Read the model definition and answer for the solid it produces. Units are mm, in the model's axes. Give positions to 0.01 mm unless a question says otherwise; leave off trailing zeros. Loops run counter-clockwise (first coordinate to the right, second up) from the corner with the lowest first, then second, coordinate; pieces in that order, holes last. Notation, with made-up numbers: (69.25, 17) - (108.25, 17) arc R20 cw to (108.25, 27) - close; hole circle Ø10 at (79, 67.25). An arc over 180 degrees is marked (long way). Write item = value, one per line.
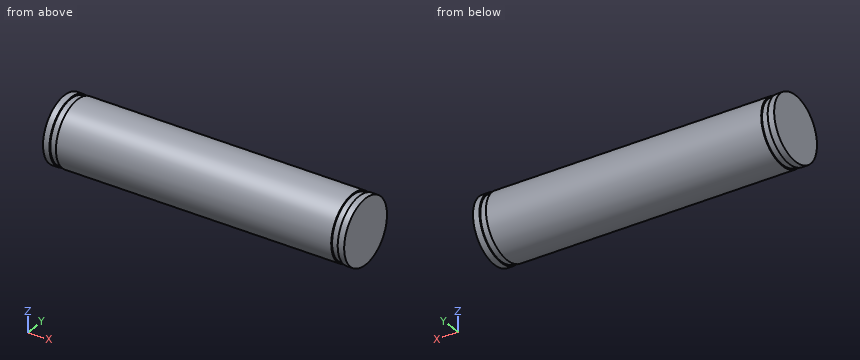
```python
from build123d import *


with BuildPart() as part:
    # Esboço1 → Revolução1 (revolve)
    with BuildSketch(Plane(origin=(0, 0, 0), x_dir=(1, 0, 0), z_dir=(0, 1, 0)), mode=Mode.PRIVATE) as revolu_o1_sk:
        Polygon((-23.25, 0), (-23.25, 5), (-22.25, 5), (-22.25, 4.8), (-21.25, 4.8), (-21.25, 5), (21.25, 5), (21.25, 4.8), (22.25, 4.8), (22.25, 5), (23.25, 5), (23.25, 0), align=None)
    revolve(revolu_o1_sk.sketch.rotate(Axis((-23.25, 0, 0), (1, 0, 0)), 180), axis=Axis((-23.25, 0, 0), (1, 0, 0)))


solid = part.part
```
1) Find the intervals of material crossed by probe 1 along Y at (x, z) = (-13, -0.25); probe 2 along Y at (x, z) = (-14.5, -1.25); probe 3 along Z at (x, y) = (-16.5, -1), in increasing order.
Output:
probe_1 = -4.99 to 4.99
probe_2 = -4.84 to 4.84
probe_3 = -4.9 to 4.9
2) A cutting plane is placed at A-A on z = -4. Determine the outline of the cut face in (x, y), then the cut area to 3 significant figures.
Output:
outline = (-23.25, -3) - (-22.25, -3) - (-22.25, -2.65) - (-21.25, -2.65) - (-21.25, -3) - (21.25, -3) - (21.25, -2.65) - (22.25, -2.65) - (22.25, -3) - (23.25, -3) - (23.25, 3) - (22.25, 3) - (22.25, 2.65) - (21.25, 2.65) - (21.25, 3) - (-21.25, 3) - (-21.25, 2.65) - (-22.25, 2.65) - (-22.25, 3) - (-23.25, 3) - close
area = 278 mm²
3) A cutting plane is placed at B-B on y = 3. Determine the outline of the cut face in (x, z), then the cut area to 3 significant figures.
Output:
outline = (-23.25, -4) - (-22.25, -4) - (-22.25, -3.75) - (-21.25, -3.75) - (-21.25, -4) - (21.25, -4) - (21.25, -3.75) - (22.25, -3.75) - (22.25, -4) - (23.25, -4) - (23.25, 4) - (22.25, 4) - (22.25, 3.75) - (21.25, 3.75) - (21.25, 4) - (-21.25, 4) - (-21.25, 3.75) - (-22.25, 3.75) - (-22.25, 4) - (-23.25, 4) - close
area = 371 mm²
4) Each of these flat-tipped pins is pushed along its axis until it touches: P1, Ø3, axis at x = -17, y = -3.5, coming from the -Z side; P2, Ø1, axis at x = -15, z = -1.5, coming from the -Y side; P3, Ø5, axis at x = -14, y = 0.5, coming from the +Z side. Where does it stop, or does it pass through?
Output:
P1 = -4.58
P2 = -4.9
P3 = 5
5) A cutting plane is placed at C-C on x = -12.5. Determine the outline of the cut face in (y, z).
Output:
outline = circle Ø10 at (0, 0)
